Could you check a few things on this model? Use its own coordinates, in mm. A direction names the side the tool comes from. Round coordinates to 2 decimals unless told otherwise and drop trailing zeros. Write each loop counter-clockwise with the first axis right and the second up, starting at its lowest first coordinate (ties: lowest second). Pieces come first, ordered by that corner, then holes. Notation, with made-up numbers: (-27, 58.25) -> (-2, 58.25) arc R31 ccw to (-2, 84.25) -> close; hole circle Ø11 at (65.5, -31). An arc over 180 degrees is marked (long way). Answer in a Markdown table with one row per item.
from build123d import *

# Parameters (mm, degrees)
F0_R     = 3.45
F1_DEPTH = 3
F2_SIZE  = 0.2
F4_DEPTH = 3
F6_COUNT = 4
F8_DEPTH = 2.3
F9_R     = 0.6


# Not quite as in the source:
# - a feature names something its author has since deleted; it is built from what else it names


with BuildPart() as f1:
    # F0 (on Top) → F1 (new body)
    with BuildSketch(Plane.XY):
        with Locations((0, 15.485)):
            Circle(F0_R)
    extrude(amount=F1_DEPTH)

    # F2
    f2_edges = [f1.edges().sort_by_distance(p)[0] for p in [
        (-3.45, 15.485, 3),
    ]]
    chamfer(f2_edges, length=F2_SIZE)

    # F3 (on face) → F4 (cut, through all)
    with BuildSketch(Plane.XY.offset(3)):
        with BuildLine():
            Line((-1, 19.435), (-1, 16.6030339887))
            ThreePointArc((-1, 16.6030339887), (-1.5, 15.485), (-1, 14.3669660113))
            Line((-1, 14.3669660113), (-1, 11.535))
            Line((-1, 11.535), (1, 11.535))
            Line((1, 11.535), (1, 14.3669660113))
            ThreePointArc((1, 14.3669660113), (1.5, 15.485), (1, 16.6030339887))
            Line((1, 16.6030339887), (1, 19.435))
            Line((1, 19.435), (-1, 19.435))
        make_face()
    extrude(amount=-F4_DEPTH, mode=Mode.SUBTRACT)


with BuildPart() as f6_1:
    # F6: instance of F1
    add(f1.part.rotate(Axis((0, 0, 1.3403603807), (0, 0, 1)), 1 * 360 / F6_COUNT))


with BuildPart() as f6_2:
    # F6: instance of F1
    add(f1.part.rotate(Axis((0, 0, 1.3403603807), (0, 0, 1)), 2 * 360 / F6_COUNT))


with BuildPart() as f6_3:
    # F6: instance of F1
    add(f1.part.rotate(Axis((0, 0, 1.3403603807), (0, 0, 1)), 3 * 360 / F6_COUNT))


with BuildPart() as f1_1:
    add(f1.part)

    add(f6_1.part)  # F8 merges F6_1

    add(f6_2.part)  # F8 merges F6_2

    add(f6_3.part)  # F8 merges F6_3
    # F7 (on Top) → F8 (join)
    with BuildSketch(Plane.XY):
        with BuildLine():
            ThreePointArc((2.3542748808, 8.4528817839), (2.5179079965, 9.995185414), (3.4299243827, 11.2496583693))
            ThreePointArc((3.4299243827, 11.2496583693), (0, 20.935), (-3.4299243827, 11.2496583693))
            ThreePointArc((-3.4299243827, 11.2496583693), (-2.5179079965, 9.995185414), (-2.3542748808, 8.4528817839))
            Line((-2.3542748808, 8.4528817839), (-3.1819805153, 3.1819805153))
            Line((-3.1819805153, 3.1819805153), (0, 4.5))
            Line((0, 4.5), (3.1819805153, 3.1819805153))
            Line((3.1819805153, 3.1819805153), (2.3542748808, 8.4528817839))
        make_face()
        Polygon((4.5, 0), (3.1819805153, 3.1819805153), (0, 4.5), (-3.1819805153, 3.1819805153), (-4.5, 0), (-3.1819805153, -3.1819805153), (0, -4.5), (3.1819805153, -3.1819805153), align=None)
        with BuildLine():
            Line((8.4528817839, 2.3542748808), (3.1819805153, 3.1819805153))
            Line((3.1819805153, 3.1819805153), (4.5, 0))
            Line((4.5, 0), (3.1819805153, -3.1819805153))
            Line((3.1819805153, -3.1819805153), (8.4528817839, -2.3542748808))
            ThreePointArc((8.4528817839, -2.3542748808), (9.995185414, -2.5179079965), (11.2496583693, -3.4299243827))
            ThreePointArc((11.2496583693, -3.4299243827), (20.935, 0), (11.2496583693, 3.4299243827))
            ThreePointArc((11.2496583693, 3.4299243827), (9.995185414, 2.5179079965), (8.4528817839, 2.3542748808))
        make_face()
        with BuildLine():
            Line((-4.5, 0), (-3.1819805153, 3.1819805153))
            Line((-3.1819805153, 3.1819805153), (-8.4528817839, 2.3542748808))
            ThreePointArc((-8.4528817839, 2.3542748808), (-9.995185414, 2.5179079965), (-11.2496583693, 3.4299243827))
            ThreePointArc((-11.2496583693, 3.4299243827), (-20.935, 0), (-11.2496583693, -3.4299243827))
            ThreePointArc((-11.2496583693, -3.4299243827), (-9.995185414, -2.5179079965), (-8.4528817839, -2.3542748808))
            Line((-8.4528817839, -2.3542748808), (-3.1819805153, -3.1819805153))
            Line((-3.1819805153, -3.1819805153), (-4.5, 0))
        make_face()
        with BuildLine():
            Line((2.3542748808, -8.4528817839), (3.1819805153, -3.1819805153))
            Line((3.1819805153, -3.1819805153), (0, -4.5))
            Line((0, -4.5), (-3.1819805153, -3.1819805153))
            Line((-3.1819805153, -3.1819805153), (-2.3542748808, -8.4528817839))
            ThreePointArc((-2.3542748808, -8.4528817839), (-2.5179079965, -9.995185414), (-3.4299243827, -11.2496583693))
            ThreePointArc((-3.4299243827, -11.2496583693), (0, -20.935), (3.4299243827, -11.2496583693))
            ThreePointArc((3.4299243827, -11.2496583693), (2.5179079965, -9.995185414), (2.3542748808, -8.4528817839))
        make_face()
    extrude(amount=-F8_DEPTH)

    # F9
    f9_edges = [f1_1.edges().sort_by_distance(p)[0] for p in [
        (2.768128, 5.817431, 0),
        (5.817431, 2.768128, 0),
        (2.517908, 9.995185, 0),
        (9.995185, 2.517908, 0),
        (0, 20.935, 0),
        (20.935, 0, 0),
        (-2.517908, 9.995185, 0),
        (9.995185, -2.517908, 0),
        (-2.768128, 5.817431, 0),
        (5.817431, -2.768128, 0),
        (-5.817431, 2.768128, 0),
        (2.768128, -5.817431, 0),
        (-9.995185, 2.517908, 0),
        (2.517908, -9.995185, 0),
        (-20.935, 0, 0),
        (0, -20.935, 0),
        (-9.995185, -2.517908, 0),
        (-2.517908, -9.995185, 0),
        (-5.817431, -2.768128, 0),
        (-2.768128, -5.817431, 0),
    ]]
    fillet(f9_edges, radius=F9_R)


solid = f1_1.part
1) Imagine slicing it at A-A, the plane z = 1.35. Count the separate pieces of the cut face and the enclosed holes in it, plus the area to 3 significant figures.
Findings:
| item | result |
|---|---|
| separate pieces | 8 |
| enclosed holes | 0 |
| area | 89.0 mm^2 |
2) For faces 4 (the face through (5.854, 2.762, -1.438)), 5 (the face through (2.63, -5.53, -0.17)), 6 (the face through (18, 1, 2)), which set-ups out of +Z, -Z, +X, -X, +Y, -Y let a thin tool reach every point of the face, with its end or its side?
Findings:
| item | result |
|---|---|
| face 4 | +Z, -Z |
| face 5 | +Z |
| face 6 | +Z, +X, -X |
3) Thinking about a two-plate mould opening in Y: for faces 1 (the face through (2, 16, 3)), 2 (the face through (18, -1, 2)), 3 (the face through (20.93, -0.19, -1.44)), which applies, +Y half, -Y half, draft (parallel to the pull), parting line (faces both ways), or undercut?
Findings:
| item | result |
|---|---|
| face 1 | draft |
| face 2 | undercut |
| face 3 | parting line |
4) For pin 1 (12 mm diameter, centred on x = -0.5, y = 0, fed in from +Z); pin 2 (3 mm diameter, centred on x = 10, z = 1, fed in from +Y); pin 3 (1.1 mm diameter, centred on x = 17.5, z = 1, fed in from -Y), each with a flat end and sliding along its axis, tell me the tip position at first contact or that it passes through.
Findings:
| item | result |
|---|---|
| pin 1 | stops at z = 0 |
| pin 2 | stops at y = 2.87 |
| pin 3 | stops at y = -3.12 |
5) Please list where these lines run through material, in increasing order: line 1 (Y direction, x = 14, z = 1.15); line 2 (X direction, y = -13, z = 1.65); line 3 (Y direction, x = 14.5, z = 0.3).
Findings:
| item | result |
|---|---|
| line 1 | y = -3.11 to -1, 1 to 3.11 |
| line 2 | x = -2.39 to -1, 1 to 2.39 |
| line 3 | y = -3.31 to -1.13, 1.13 to 3.31 |
6) Imagine slicing it at B-B, the plane x = 0. Please give me the cut outline in (y, z) (3 decimals).
Findings:
| item | result |
|---|---|
| outline | (-20.935, -2.3) -> (20.935, -2.3) -> (20.935, -0.6) arc R0.6 ccw to (20.335, 0) -> (-20.335, 0) arc R0.6 ccw to (-20.935, -0.6) -> close |
